Can you work these out from the model? Positions are in its coordinate system, mm. Round coordinates to 2 decimals unless told otherwise and drop trailing zeros. Write each loop counter-clockwise with the first axis right and the second up, starting at its lowest first coordinate (ties: lowest second). Pieces come first, ordered by that corner, then holes. Notation, with made-up numbers: (20, -28.75) - (25, -28.75) arc R31 ccw to (25, 5.25) - close; hole circle Ø7 at (49, 16). An arc over 180 degrees is marked (long way). One line per item, written item: value. Start each with the question number.
(1) If I drill on L1, parallel to Z at x = 53.5, y = -57.5; L2, parallel to Z at x = 172.5, y = -168; L3, parallel to Y at x = 228.5, z = -14.5, over which ranges is the centre line in solid material (lowest first)? Write a range as from..to.
(2) I want a section at B-B on x = 86.5. List the corners of the cut face in (y, z) for me.
(3) I'm going to push flat-ended pins straight in: pin 1 Ø6 at (x, z) = (150.5, 120.5) entering from +Y; pin 2 Ø5 at (x, z) = (122.5, 115) entering from -Y; pin 3 Ø8 at (x, z) = (128.5, 132.5) entering from +Y. Where does each tip first touch, or does it pass through?
(4) I want a section at A-A on y = -110. List the corners of the cut face in (x, z) for me, plus the area to 3 significant figures.
(5) I want a section at C-C on z = 154. List the corners of the cut face in (x, y) for me, plus the area to 3 significant figures.
(6) I want a section at D-D on z = -61.5. List the corners of the cut face in (x, y) for me, plus the area to 3 significant figures.
from build123d import *

# Parameters (mm, degrees)
F0_W       = 304.8
F0_H       = 304.8
F1_DEPTH   = 95.25
F1_FACE_W  = 304.8
F1_FACE_H  = 304.8
F2_DEPTH   = 101.6
F2_TAPER   = 57
F1_FACE1_W = 304.8
F1_FACE1_H = 304.8


# Not quite as in the source:
# - an extrude whose draft closes it to a point is written as a loft to that point


with BuildPart() as f1:
    # F0 (on Top) → F1 (new body)
    with BuildSketch(Plane.XY):
        with Locations((152.4, -152.4)):
            Rectangle(F0_W, F0_H)
    extrude(amount=F1_DEPTH)

    # F1_face (on face) → F2 (join)
    with BuildSketch(Plane(origin=(152.4, -152.4, 95.25), x_dir=(1, 0, 0), z_dir=(0, 0, 1))):
        Rectangle(F1_FACE_W, F1_FACE_H)
    extrude(amount=F2_DEPTH, taper=F2_TAPER)

    # F1_face1 (on face) → F3 section 0
    with BuildSketch(Plane(origin=(152.4, -152.4, 0), x_dir=(1, 0, 0), z_dir=(0, 0, -1)), mode=Mode.PRIVATE) as f3_s0:
        Rectangle(F1_FACE1_W, F1_FACE1_H)
    loft([f3_s0.sketch, Vertex(152.4, -152.4, -98.9697172033)], ruled=True)


solid = f1.part
Established:
1. L1: -34.74..129.99
1. L2: -85.92..181.17
1. L3: -282.47..-22.33
2. outline: (-304.8, 0) - (-218.3, -56.17) - (-86.5, -56.17) - (0, 0) - (0, 95.25) - (-86.5, 151.42) - (-218.3, 151.42) - (-304.8, 95.25) - close
3. pin 1: y = -34.26
3. pin 2: y = -278.24
3. pin 3: y = -51.2
4. outline: (0, 0) - (110, -71.43) - (194.8, -71.43) - (304.8, 0) - (304.8, 95.25) - (194.8, 166.68) - (110, 166.68) - (0, 95.25) - close
4. area: 56,900 mm2
5. outline: (90.47, -214.33) - (214.33, -214.33) - (214.33, -90.47) - (90.47, -90.47) - close
5. area: 15,300 mm2
6. outline: (94.7, -210.1) - (210.1, -210.1) - (210.1, -94.7) - (94.7, -94.7) - close
6. area: 13,300 mm2
